from build123d import *

# Parameters (mm, degrees)
SKETCH1_W           = 114.3
SKETCH1_H           = 66.675
SKETCH1_R           = 1.016
SKETCH1_W_2         = 1.5875
SKETCH1_H_2         = 20.0000108
BOSS_EXTRUDE1_DEPTH = 3.175
SKETCH2_W           = 10.16
SKETCH2_H           = 3.175
BOSS_EXTRUDE3_DEPTH = 3.175
CUT_EXTRUDE1_DEPTH  = 3.175


with BuildPart() as part:
    # Sketch1 → Boss-Extrude1 (new body)
    with BuildSketch(Plane(origin=(0, 0, 0), x_dir=(1, 0, 0), z_dir=(0, 1, 0))):
        with Locations((57.15, 33.3375)):
            Rectangle(SKETCH1_W, SKETCH1_H)
        with Locations((1.905, 15.5575)):
            Circle(SKETCH1_R, mode=Mode.SUBTRACT)
        with Locations((23.495, 15.5575)):
            Circle(SKETCH1_R, mode=Mode.SUBTRACT)
        with Locations((23.495, 51.1175)):
            Circle(SKETCH1_R, mode=Mode.SUBTRACT)
        with Locations((1.905, 51.1175)):
            Circle(SKETCH1_R, mode=Mode.SUBTRACT)
        with Locations((110.96625, 33.3375)):
            Rectangle(SKETCH1_W_2, SKETCH1_H_2, mode=Mode.SUBTRACT)
        with Locations((62.55385, 33.3375)):
            Rectangle(SKETCH1_W_2, SKETCH1_H_2, mode=Mode.SUBTRACT)
    extrude(amount=BOSS_EXTRUDE1_DEPTH)

    # Sketch2 → Boss-Extrude3 (add)
    with BuildSketch(Plane.XY):
        with Locations((40.770613131, 1.5875)):
            Rectangle(SKETCH2_W, SKETCH2_H)
        with Locations((61.090613131, 1.5875)):
            Rectangle(SKETCH2_W, SKETCH2_H)
    boss_extrude3 = extrude(amount=BOSS_EXTRUDE3_DEPTH)

    # Mirror2: Boss-Extrude3 across plane
    add(boss_extrude3.mirror(Plane(origin=(0, 3.175, -33.3375), x_dir=(1, 0, 0), z_dir=(0, 0, -1))))

    # Sketch4 → Cut-Extrude1 (cut)
    with BuildSketch(Plane(origin=(0, 3.175, 0), x_dir=(1, 0, 0), z_dir=(0, 1, 0))):
        Polygon((28.705613131, 0), (28.705613131, 2.54), (26.800613131, 2.54), (26.800613131, 5.73532), (28.705613131, 5.73532), (28.705613131, 7.64032), (32.515613131, 7.64032), (32.515613131, 5.73532), (34.420613131, 5.73532), (34.420613131, 2.54), (32.515613131, 2.54), (32.515613131, 0), align=None)
        Polygon((49.025613131, 0), (49.025613131, 2.54), (47.120613131, 2.54), (47.120613131, 5.73532), (49.025613131, 5.73532), (49.025613131, 7.64032), (52.835613131, 7.64032), (52.835613131, 5.73532), (54.740613131, 5.73532), (54.740613131, 2.54), (52.835613131, 2.54), (52.835613131, 0), align=None)
        Polygon((52.835613131, 66.675), (52.835613131, 64.135), (54.740613131, 64.135), (54.740613131, 60.93968), (52.835613131, 60.93968), (52.835613131, 59.03468), (49.025613131, 59.03468), (49.025613131, 60.93968), (47.120613131, 60.93968), (47.120613131, 64.135), (49.025613131, 64.135), (49.025613131, 66.675), align=None)
        Polygon((32.515613131, 66.675), (32.515613131, 64.135), (34.420613131, 64.135), (34.420613131, 60.93968), (32.515613131, 60.93968), (32.515613131, 59.03468), (28.705613131, 59.03468), (28.705613131, 60.93968), (26.800613131, 60.93968), (26.800613131, 64.135), (28.705613131, 64.135), (28.705613131, 66.675), align=None)
    extrude(amount=-CUT_EXTRUDE1_DEPTH, mode=Mode.SUBTRACT)


solid = part.part
Here's how the part is built. I have some questions about the finished solid (model axes, mm). A direction names the side the tool comes from. Round coordinates to 2 decimals unless told otherwise and drop trailing zeros. Write each loop counter-clockwise with the first axis right and the second up, starting at its lowest first coordinate (ties: lowest second). Pieces come first, ordered by that corner, then holes.
1. For faces 1 (the flat face through (28.706, 2, -65)), 2 (the flat face through (47.121, 2, -4)), 3 (the flat face through (51, 2, -7.64)), which set-ups out of +Z, -Z, +X, -X, +Y, -Y let a thin tool reach every point of the face, with its end or its side?
2. I need wall thicknesses on L1, parallel to X at y = 1.3, z = -59.5; L2, parallel to X at y = 1.45, z = -3; L3, parallel to X at y = 0.65, z = 0.5. Which ranges of each line are inside material? Lowest first, please.
3. Suppose I cut it at C-C (y = 2). State how many separate pieces and enclosed holes the cut face has, and give its area (3 significant figures).
4. If we mould it in two halves opening along Z, with no side actions, what happens to faces 4 (the flat face through (34.421, 2, -4)), 5 (the flat face through (56, 3.175, -34)), 6 (the flat face through (47, 2, 0))? For each: released by +Z, released by -Z, zero draft, split by the parting line, or undercut.
5. Will these pins go through, and if not, where does the flat tip stop? pin 1 Ø0.6 at (x, y) = (48, 1.5) entering from +Z; pin 2 Ø1 at (x, y) = (33, 1.5) entering from -Z (3 decimals); pin 3 Ø1 at (y, z) = (2, -60.5) entering from -X; pin 4 Ø1 at (y, z) = (1.5, 1.5) entering from +X.
6. Suppose I cut it at A-A (z = -28). List the corners of the cut face in (x, y) for me (1 decimal).
7. Suppose I cut it at B-B (x = 86.5). List the corners of the cut face in (y, z) for me (3 decimals), and give its area (3 significant figures).
Answer sheet:
1. face 1: -Z, +Y, -Y
1. face 2: +Y, -Y
1. face 3: +Z, +Y, -Y
2. L1: x = 0 to 28.71, 32.52 to 49.03, 52.84 to 114.3
2. L2: x = 0 to 26.8, 34.42 to 47.12, 54.74 to 114.3
2. L3: x = 35.69 to 45.85, 56.01 to 66.17
3. separate pieces: 1
3. enclosed holes: 6
3. area: 7,510 mm2
4. face 4: undercut
4. face 5: zero draft
4. face 6: released by +Z
5. pin 1: stops at z = 0
5. pin 2: stops at z = -66.675
5. pin 3: stops at x = 0
5. pin 4: stops at x = 66.17
6. outline: (0, 0) - (61.8, 0) - (61.8, 3.2) - (0, 3.2) - close; (63.3, 0) - (110.2, 0) - (110.2, 3.2) - (63.3, 3.2) - close; (111.8, 0) - (114.3, 0) - (114.3, 3.2) - (111.8, 3.2) - close
7. outline: (0, -66.675) - (3.175, -66.675) - (3.175, 0) - (0, 0) - close
7. area: 212 mm2
